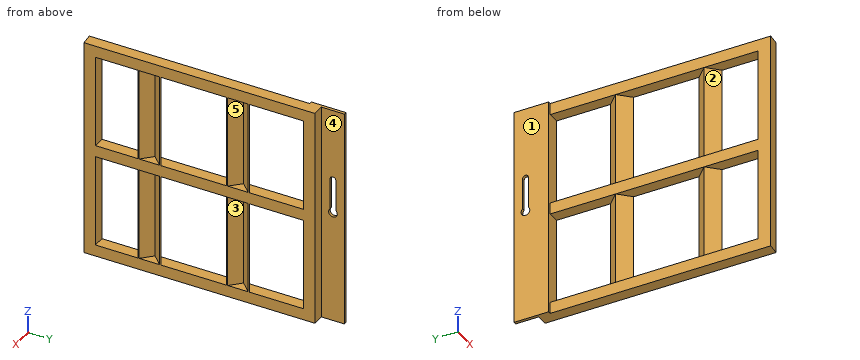
```python
from build123d import *

# Parameters (mm, degrees)
F0_W     = 25.4
F0_H     = 25.4
F0_W_2   = 21.1836
F0_H_2   = 21.1836
F1_DEPTH = 508
F2_W     = 25.4
F2_H     = 25.4
F3_DEPTH = 482.6
F4_W     = 76.2
F4_H     = 482.6
F5_DEPTH = 6.35
F7_DEPTH = 482.6
F9_DEPTH = 482.6


with BuildPart() as f1:
    # F0 (on Front) → F1 (new body)
    with BuildSketch(Plane.XZ):
        with Locations((0, 457.2)):
            Rectangle(F0_W, F0_H)
        with Locations((0, 457.2)):
            Rectangle(F0_W_2, F0_H_2, mode=Mode.SUBTRACT)
        with Locations((0, 228.6)):
            Rectangle(F0_W, F0_H)
        with Locations((0, 228.6)):
            Rectangle(F0_W_2, F0_H_2, mode=Mode.SUBTRACT)
        Rectangle(F0_W, F0_H)
        Rectangle(F0_W_2, F0_H_2, mode=Mode.SUBTRACT)
    extrude(amount=F1_DEPTH)

    # F2 (on face) → F3 (join)
    with BuildSketch(Plane.XY.offset(469.9)):
        with Locations((0, -12.7)):
            Rectangle(F2_W, F2_H)
        with Locations((0, -495.3)):
            Rectangle(F2_W, F2_H)
    extrude(amount=-F3_DEPTH)

    # F4 (on face) → F5 (join)
    with BuildSketch(Plane(origin=(-12.7, 0, 0), x_dir=(0, -1, 0), z_dir=(-1, 0, 0))):
        with Locations((-12.7, 228.6)):
            Rectangle(F4_W, F4_H)
        with BuildLine():
            ThreePointArc((-19.05, 242.049516), (-25.4, 225.425), (-31.75, 242.049516))
            Line((-31.75, 242.049516), (-31.75, 311.15))
            ThreePointArc((-31.75, 311.15), (-25.4, 317.5), (-19.05, 311.15))
            Line((-19.05, 311.15), (-19.05, 242.049516))
        make_face(mode=Mode.SUBTRACT)
    extrude(amount=F5_DEPTH)

    # F6 (on face) → F7 (join)
    with BuildSketch(Plane.XY.offset(469.9)):
        Polygon((-12.7, -169.333333), (12.7, -194.733333), (12.7, -191.751888), (-9.718555, -169.333333), (12.7, -146.914778), (12.7, -143.933333), align=None)
        Polygon((-12.7, -364.066667), (12.7, -389.466667), (12.7, -386.485222), (-9.718555, -364.066667), (12.7, -341.648112), (12.7, -338.666667), align=None)
    extrude(amount=-F7_DEPTH)

    # F8 (on face) → F9 (join)
    with BuildSketch(Plane.XY.offset(469.9)):
        Polygon((-12.7, -510.38125), (12.7, -508), (-12.7, -508), align=None)
    extrude(amount=-F9_DEPTH)


solid = f1.part
```
The listing builds one solid part. Answer for the finished solid, in the listing's coordinates (mm). Face numbers are marked on the shaded views. A direction names the side the tool comes from. Coordinates: 2 decimals unless noted, no trailing zeros. Loops run counter-clockwise (first coordinate to the right, second up) from the corner with the lowest first, then second, coordinate; pieces in that order, holes last. Notation, with made-up numbers: M -11,59 L 15,59 A17 cw 15,88 Z; hole C 52.25,3 d2. An arc over 180 degrees is marked long. Answer as CSV lines item,"result". Start each with the question number.
(1) Given pin 1 (6.5 mm diameter, centred on x = 0.5, z = 452, fed in from -Y); pin 2 (3 mm diameter, centred on x = -4.5, z = 106, fed in from +Y); pin 3 (3 mm diameter, centred on x = 0.5, z = 104, fed in from -Y); pin 4 (12 mm diameter, centred on x = -8.5, z = 333.5, fed in from +Y), each flat-ended and moving along its own axis, determine where each tip first touches the part or whether it passes through.
(2) The part is cut by section C-C (z = 395). Give the vertices of the cut face in (x, y), and give its area (3 significant figures).
(3) For the marked faces 1, 2 and 3, determine the directions among +Z, -Z, +X, -X, +Y, -Y from which every point of the face is accessible in a straight line to the end or side of a thin tool.
(4) The mould has two halves that part along Y. Classify the marked faces 4 and 5: pulls with the +Y half, pulls with the -Y half, needs draft (parallel to the pull), parting line crosses it, or undercut.
(5) The part is cut by section D-D (x = 1). State how many separate pieces and enclosed holes the cut face has, and give its area (3 significant figures).
(6) The part is cut by section B-B (y = 25.4). Give the vertices of the cut face in (x, z) (3 decimals), and give its area (3 significant figures).
(7) The part is cut by section A-A (y = -57). Give the vertices of the cut face in (x, z).
(8) Find the intervals of material crossed by L1, parallel to Z at x = -2, y = -410; L2, parallel to Y at x = -12, z = 274; L3, parallel to Y at x = -15, z = 234, in increasing order. Write a range as [from, to].
Determined:
1,pin 1,"y = -509.45"
1,pin 2,"y = 0"
1,pin 3,"y = -509.28"
1,pin 4,"y = 50.8"
2,outline,"M -19.05,-25.4 L 12.7,-25.4 L 12.7,0 L -12.7,0 L -12.7,50.8 L -19.05,50.8 Z; M -12.7,-510.38 L 12.7,-508 L 12.7,-482.6 L -12.7,-482.6 Z; M -12.7,-364.07 L 12.7,-389.47 L 12.7,-386.49 L -9.72,-364.07 L 12.7,-341.65 L 12.7,-338.67 Z; M -12.7,-169.33 L 12.7,-194.73 L 12.7,-191.75 L -9.72,-169.33 L 12.7,-146.91 L 12.7,-143.93 Z"
2,area,"2,090 mm2"
3,face 1,"+Z, -Z, -X, +Y, -Y"
3,face 2,"-X"
3,face 3,"+X"
4,face 4,"needs draft"
4,face 5,"undercut"
5,separate pieces,"1"
5,enclosed holes,"25"
5,area,"36,400 mm2"
6,outline,"M -19.05,-12.7 L -12.7,-12.7 L -12.7,225.425 L -19.05,225.425 Z; M -19.05,317.5 L -12.7,317.5 L -12.7,469.9 L -19.05,469.9 Z"
6,area,"2,480 mm2"
7,outline,"M -12.7,-12.7 L 12.7,-12.7 L 12.7,12.7 L -12.7,12.7 Z; M -12.7,215.9 L 12.7,215.9 L 12.7,241.3 L -12.7,241.3 Z; M -12.7,444.5 L 12.7,444.5 L 12.7,469.9 L -12.7,469.9 Z; hole M -10.59,-10.59 L 10.59,-10.59 L 10.59,10.59 L -10.59,10.59 Z; hole M -10.59,218.01 L 10.59,218.01 L 10.59,239.19 L -10.59,239.19 Z; hole M -10.59,446.61 L 10.59,446.61 L 10.59,467.79 L -10.59,467.79 Z"
8,L1,"[-12.7, -10.59], [10.59, 12.7], [215.9, 218.01], [239.19, 241.3], [444.5, 446.61], [467.79, 469.9]"
8,L2,"[-510.32, -482.6], [-364.77, -363.37], [-170.03, -168.63], [-25.4, 0]"
8,L3,"[-25.4, 15.92], [34.88, 50.8]"
